Model file for the job. Use its own axes, mm. A direction names the side the tool comes from. Give positions to 0.01 mm unless a question says otherwise; leave off trailing zeros. Order: outer loops, then holes, each group sorted by start corner. A loop starts at its lowest first (then second) coordinate and runs counter-clockwise, first axis right, second up. Notation, with made-up numbers: (0, -21.75) -> (44, -21.75) arc R23 ccw to (44, 4.25) -> close; hole circle Ø9 at (67, 42.5). An arc over 180 degrees is marked (long way). Use CSV: the item, a comma, the result in double quotes. Start each with the question number.
1. 3-axis set-ups, long thin cutter, end or side, ignore diameter. For faces 4 (the flat face through (-30, 17.082, 5)), 5 (the cylindrical face through (-17.24, -20.1, 5.03)), 6 (the flat face through (-18.1, -12, 2)), 7 (the flat face through (-15.1, 0, 9)): which of +Z, -Z, +X, -X, +Y, -Y reach the whole face in a straight line?
2. Pull direction X, two halves, no side cores. Call faces 1 (the flat face through (0, -21, 5)), 2 (the flat face through (-43.1, 11, 5)), 3 (the flat face through (0, -18.5, 5)): released by +X, released by -X, zero draft, split by the parting line, or undercut.
3. Cut at C-C on y = -2.5. List the corners of the cut face in (x, z), then the cut area to 3 significant figures.
4. Drop flat-ended pins along their axis: pin 1 (4.5 mm diameter, centred on x = -33, z = 4, fed in from +Y); pin 2 (2 mm diameter, centred on x = -35, z = 6, fed in from -Y); pin 3 (1.2 mm diameter, centred on y = 0, z = 4.5, fed in from -X). Give the stop position or say it passes through.
5. Cut at D-D on x = -31.5. List the corners of the cut face in (y, z), then the cut area to 3 significant figures.
6. Wall check: line 1 (Y direction, x = -8, z = 6.75); line 2 (X direction, y = 1.5, z = 3); line 3 (X direction, y = -14, z = 9). Give the ranges that are in metal, low to high. Write a range as from..to.
7. Cut at B-B on y = 8. List the corners of the cut face in (x, z), then the cut area to 3 significant figures.
8. Cut at A-A on x = 10. List the corners of the cut face in (y, z).
```python
from build123d import *

# Parameters (mm, degrees)
F0_W     = 36.2
F0_H     = 42
F1_DEPTH = 10
F2_R     = 3
F3_T     = -2.5
F5_DEPTH = 3
F6_R     = 1
F7_W     = 12.1205560863
F7_H     = 4
F8_DEPTH = 25


# Not quite as in the source:
# - a shell that OpenCascade refuses in one call is made with other operations: the cavity is built on its own and cut out


with BuildPart() as f1:
    # F0 (on Top) → F1 (new body)
    with BuildSketch(Plane.XY):
        Rectangle(F0_W, F0_H)
    extrude(amount=F1_DEPTH)

    # F2
    f2_edges = [f1.edges().sort_by_distance(p)[0] for p in [
        (-18.1, -21, 5),
        (18.1, -21, 5),
        (0, -21, 0),
        (0, -21, 10),
        (-18.1, 21, 5),
        (-18.1, 0, 0),
        (-18.1, 0, 10),
        (18.1, 21, 5),
        (0, 21, 0),
        (0, 21, 10),
        (18.1, 0, 0),
        (18.1, 0, 10),
    ]]
    fillet(f2_edges, radius=F2_R)

    # F3: a shell. OpenCascade refuses it in one call, so the cavity is built on its own and cut out:
    # the body offset inwards by the wall thickness, plus a prism from it out through each open face.
    f3_core = offset(f1.part, amount=F3_T, mode=Mode.PRIVATE)
    f3_exits = [f3_core.faces().sort_by_distance(p)[0] for p in [
        (0, 0, 7.5),
    ]]
    add(f3_core, mode=Mode.SUBTRACT)
    extrude(f3_exits, amount=-F3_T, mode=Mode.SUBTRACT)

    # F4 (on face) → F5 (join)
    with BuildSketch(Plane(origin=(-18.1, 0, 0), x_dir=(0, -1, 0), z_dir=(-1, 0, 0))):
        with BuildLine():
            ThreePointArc((7.0906764033, 3), (11.6732520983, 0), (16.2558277932, 3))
            Line((16.2558277932, 3), (7.0906764033, 3))
        make_face()
        with BuildLine():
            Line((7.0906764033, 7), (16.2558277932, 7))
            ThreePointArc((16.2558277932, 7), (11.6732520983, 10), (7.0906764033, 7))
        make_face()
        with BuildLine():
            ThreePointArc((16.2558277932, 3), (16.5677836629, 3.9784517816), (16.6732520983, 5))
            ThreePointArc((16.6732520983, 5), (16.5677836629, 6.0215482184), (16.2558277932, 7))
            Line((16.2558277932, 7), (7.0906764033, 7))
            ThreePointArc((7.0906764033, 7), (6.6732520983, 5), (7.0906764033, 3))
            Line((7.0906764033, 3), (16.2558277932, 3))
        make_face()
    extrude(amount=F5_DEPTH)

    # F6
    f6_edges = [f1.edges().sort_by_distance(p)[0] for p in [
        (-21.1, -7.090676, 7),
    ]]
    fillet(f6_edges, radius=F6_R)

    # F7 (on face) → F8 (join)
    with BuildSketch(Plane(origin=(-18.1, 0, 0), x_dir=(0, -1, 0), z_dir=(-1, 0, 0))):
        with Locations((-11.0213514417, 5)):
            Rectangle(F7_W, F7_H)
    extrude(amount=F8_DEPTH)


solid = f1.part
```
Verdict:
1,face 4,"+Z, -Z, -X, +Y"
1,face 5,"+Z, -Z, -X, -Y"
1,face 6,"none"
1,face 7,"+Z"
2,face 1,"zero draft"
2,face 2,"released by -X"
2,face 3,"undercut"
3,outline,"(-18.1, 3) arc R3 ccw to (-15.1, 0) -> (15.1, 0) arc R3 ccw to (18.1, 3) -> (18.1, 7) arc R3 ccw to (15.1, 10) -> (15.1, 7.5) arc R0.5 cw to (15.6, 7) -> (15.6, 3) arc R0.5 cw to (15.1, 2.5) -> (-15.1, 2.5) arc R0.5 cw to (-15.6, 3) -> (-15.6, 7) arc R0.5 cw to (-15.1, 7.5) -> (-15.1, 10) arc R3 ccw to (-18.1, 7) -> close"
3,area,"123 mm^2"
4,pin 1,"y = 17.08"
4,pin 2,"y = 4.96"
4,pin 3,"x = -18.1"
5,outline,"(4.96, 3) -> (17.08, 3) -> (17.08, 7) -> (4.96, 7) -> close"
5,area,"48.5 mm^2"
6,line 1,"-21..-18.5, 18.5..21"
6,line 2,"-18.1..-15.6, 15.6..18.1"
6,line 3,"-20.88..-18.1, -17.34..-15.1, 15.1..17.34"
7,outline,"(-43.1, 3) -> (-18.1, 3) arc R3 ccw to (-15.1, 0) -> (15.1, 0) arc R3 ccw to (18.1, 3) -> (18.1, 7) arc R3 ccw to (15.1, 10) -> (15.1, 7.5) arc R0.5 cw to (15.6, 7) -> (15.6, 3) arc R0.5 cw to (15.1, 2.5) -> (-15.1, 2.5) arc R0.5 cw to (-15.6, 3) -> (-15.6, 7) arc R0.5 cw to (-15.1, 7.5) -> (-15.1, 10) arc R3 ccw to (-18.1, 7) -> (-43.1, 7) -> close"
7,area,"223 mm^2"
8,outline,"(-21, 3) arc R3 ccw to (-18, 0) -> (18, 0) arc R3 ccw to (21, 3) -> (21, 7) arc R3 ccw to (18, 10) -> (18, 7.5) arc R0.5 cw to (18.5, 7) -> (18.5, 3) arc R0.5 cw to (18, 2.5) -> (-18, 2.5) arc R0.5 cw to (-18.5, 3) -> (-18.5, 7) arc R0.5 cw to (-18, 7.5) -> (-18, 10) arc R3 ccw to (-21, 7) -> close"
